from build123d import *

# Parameters (mm, degrees)
SKETCH1_W               = 46
SKETCH1_H               = 31
SKETCH1_R               = 2
BOSS_EXTRUDE1_DEPTH     = 10
FILLET1_R               = 10
BOSS_EXTRUDE2_START     = 15.5
BOSS_EXTRUDE2_DEPTH     = 10
BOSS_EXTRUDE3_START     = -15.5
BOSS_EXTRUDE3_DEPTH     = 10
SKETCH4_W               = 40
SKETCH4_H               = 5
CUT_EXTRUDE1_DEPTH      = 30.483045976
CUT_EXTRUDE1_DEPTH_BACK = 30.483045976
FILLET2_R               = 2


with BuildPart() as part:
    # Sketch1 → Boss-Extrude1 (new body)
    with BuildSketch(Plane.XY):
        Rectangle(SKETCH1_W, SKETCH1_H)
        with Locations((-15, 7.5)):
            Circle(SKETCH1_R, mode=Mode.SUBTRACT)
        with Locations((15, 7.5)):
            Circle(SKETCH1_R, mode=Mode.SUBTRACT)
        with Locations((15, -7.5)):
            Circle(SKETCH1_R, mode=Mode.SUBTRACT)
        with Locations((-15, -7.5)):
            Circle(SKETCH1_R, mode=Mode.SUBTRACT)
    extrude(amount=BOSS_EXTRUDE1_DEPTH)

    # Fillet1
    fillet1_edges = [part.edges().sort_by_distance(p)[0] for p in [
        (23, -15.5, 5),
        (-23, -15.5, 5),
        (-23, 15.5, 5),
        (23, 15.5, 5),
    ]]
    fillet(fillet1_edges, radius=FILLET1_R)

    # Sketch3 → Boss-Extrude2 (add)
    with BuildSketch(Plane(origin=(0, 0, 0), x_dir=(1, 0, 0), z_dir=(0, 1, 0)).offset(BOSS_EXTRUDE2_START)):
        with BuildLine():
            Line((-5, 3.708712153), (-5, 0))
            Line((-5, 0), (5, 0))
            Line((5, 0), (5, 3.708712153))
            ThreePointArc((5, 3.708712153), (0, 0.5), (-5, 3.708712153))
        make_face()
    extrude(amount=-BOSS_EXTRUDE2_DEPTH)

    # Sketch3<3> → Boss-Extrude3 (add)
    with BuildSketch(Plane(origin=(0, 0, 0), x_dir=(1, 0, 0), z_dir=(0, 1, 0)).offset(BOSS_EXTRUDE3_START)):
        with BuildLine():
            Line((-5, 3.708712153), (-5, 0))
            Line((-5, 0), (5, 0))
            Line((5, 0), (5, 3.708712153))
            ThreePointArc((5, 3.708712153), (0, 0.5), (-5, 3.708712153))
        make_face()
    extrude(amount=BOSS_EXTRUDE3_DEPTH)

    # Sketch4 → Cut-Extrude1 (cut, two sides)
    with BuildSketch(Plane(origin=(0, 0, 0), x_dir=(-1, 0, 0), z_dir=(0, 0, -1))) as cut_extrude1_sk:
        Rectangle(SKETCH4_W, SKETCH4_H)
    extrude(amount=CUT_EXTRUDE1_DEPTH, mode=Mode.SUBTRACT)
    extrude(cut_extrude1_sk.sketch, amount=-CUT_EXTRUDE1_DEPTH_BACK, mode=Mode.SUBTRACT)

    # Fillet2
    fillet2_edges = [part.edges().sort_by_distance(p)[0] for p in [
        (-20, 2.5, 5),
        (-20, -2.5, 5),
        (20, -2.5, 5),
        (20, 2.5, 5),
    ]]
    fillet(fillet2_edges, radius=FILLET2_R)


solid = part.part
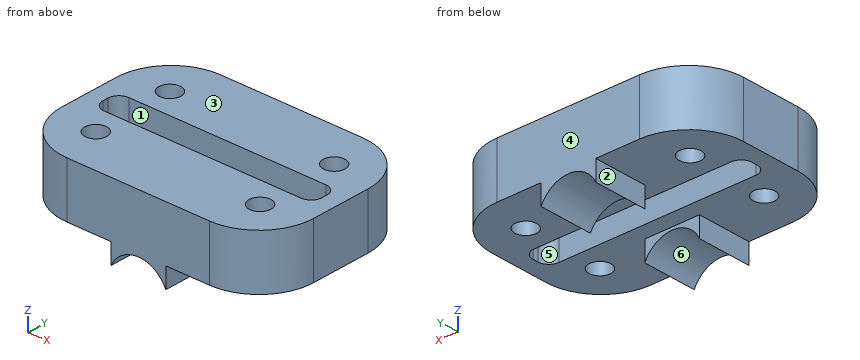
Can you work these out from the model? Positions are in its coordinate system, mm. Face numbers are marked on the shaded views. A direction names the side the tool comes from. Give positions to 0.01 mm unless a question says otherwise; leave off trailing zeros. Loops run counter-clockwise (first coordinate to the right, second up) from the corner with the lowest first, then second, coordinate; pieces in that order, holes last. Notation, with made-up numbers: (22.25, -7) - (81.25, -7) arc R36 ccw to (81.25, 32) - close; hole circle Ø8 at (53.5, 75.5). An arc over 180 degrees is marked (long way). Return JSON: item names as keys, results as strings.
1. I want a section at B-B on y = 7.5. Please give me the cut outline in (x, z).
Output values:
{"outline": "(-22.8, 0) - (-17, 0) - (-17, 10) - (-22.8, 10) - close; (-13, 0) - (-5, 0) - (-5, -3.71) arc R5.5 cw to (5, -3.71) - (5, 0) - (13, 0) - (13, 10) - (-13, 10) - close; (17, 0) - (22.8, 0) - (22.8, 10) - (17, 10) - close"}
2. For the marked faces 1, 2 and 3, which set-ups out of +Z, -Z, +X, -X, +Y, -Y let a thin tool reach every point of the face, with its end or its side?
Output values:
{"face 1": "+Z, -Z", "face 2": "-Z, -X, +Y, -Y", "face 3": "+Z, +X, -X, +Y, -Y"}
3. We'd pull the mould along Y, two halves only. Please class the marked faces 4, 5 and 6: +Y half, -Y half, draft (parallel to the pull), parting line (faces both ways), or undercut.
Output values:
{"face 4": "+Y half", "face 5": "undercut", "face 6": "draft"}
4. I want a section at C-C on z = 4. Please give me the cut outline in (x, y), and give its area (3 significant figures).
Output values:
{"outline": "(-23, -5.5) arc R10 ccw to (-13, -15.5) - (13, -15.5) arc R10 ccw to (23, -5.5) - (23, 5.5) arc R10 ccw to (13, 15.5) - (-13, 15.5) arc R10 ccw to (-23, 5.5) - close; hole (-20, -0.5) arc R2 ccw to (-18, -2.5) - (18, -2.5) arc R2 ccw to (20, -0.5) - (20, 0.5) arc R2 ccw to (18, 2.5) - (-18, 2.5) arc R2 ccw to (-20, 0.5) - close; hole circle Ø4 at (-15, -7.5); hole circle Ø4 at (-15, 7.5); hole circle Ø4 at (15, -7.5); hole circle Ø4 at (15, 7.5)", "area": "1,090 mm²"}
5. I'm going to push flat-ended pins straight in: pin 1 Ø1.5 at (y, z) = (10.5, 1) entering from -X; pin 2 Ø1.5 at (y, z) = (7.5, 4) entering from -X; pin 3 Ø4.5 at (x, y) = (-15, -7.5) entering from -Z; pin 4 Ø3 at (x, y) = (-15, 7.5) entering from -Z. Where does each tip first touch, or does it pass through?
Output values:
{"pin 1": "stops at x = -22.05", "pin 2": "stops at x = -22.92", "pin 3": "stops at z = 0", "pin 4": "passes through"}
6. I want a section at A-A on x = 9.5. Please give me the cut outline in (y, z), and give its area (3 significant figures).
Output values:
{"outline": "(-15.5, 0) - (-2.5, 0) - (-2.5, 10) - (-15.5, 10) - close; (2.5, 0) - (15.5, 0) - (15.5, 10) - (2.5, 10) - close", "area": "260 mm²"}
7. I want a section at D-D on y = 1.5. Please give me the cut outline in (x, z), and give its area (3 significant figures).
Output values:
{"outline": "(-23, 0) - (-19.73, 0) - (-19.73, 10) - (-23, 10) - close; (19.73, 0) - (23, 0) - (23, 10) - (19.73, 10) - close", "area": "65.4 mm²"}
8. If I drill on line 1 (Y direction, x = -15, z = 5.75); line 2 (Y direction, x = 0.5, z = 5.75); line 3 (X direction, y = 0, z = 7.75), over which ranges is the centre line in solid material (lowest first)?
Output values:
{"line 1": "y = -15.3 to -9.5, -5.5 to -2.5, 2.5 to 5.5, 9.5 to 15.3", "line 2": "y = -15.5 to -2.5, 2.5 to 15.5", "line 3": "x = -23 to -20, 20 to 23"}
